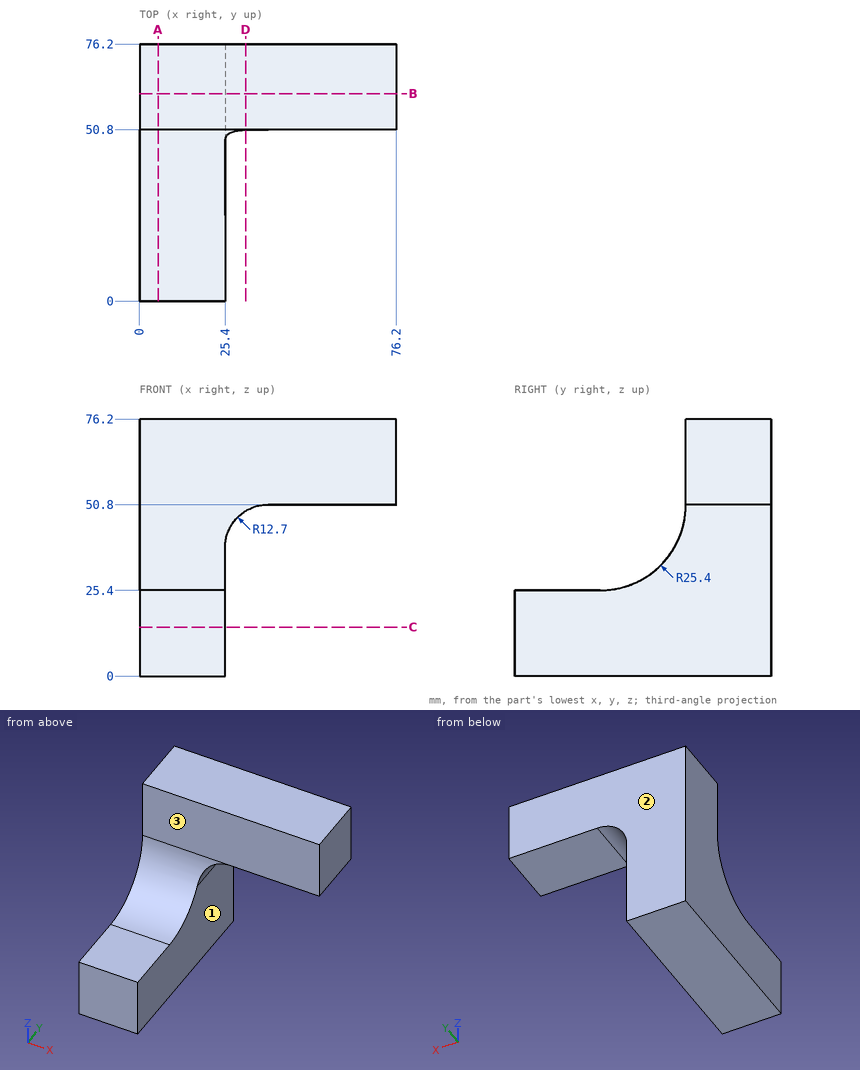
Answer from the drawing. Dimensions are ordinates in mm from the lowest x, y and z of the part. A direction names the side the tool comes from. Give positions to 0.01 mm unless a question says otherwise; leave off trailing zeros. Order: outer loops, then holes, each group sorted by start corner. A loop starts at its lowest first (then second) coordinate and runs counter-clockwise, first axis right, second up.
(1) Find section A-A (x = 5.5). Give the vertices of the cut face in (y, z), plus the area to 3 significant figures.
(2) For the marked faces 1, 2 and 3, determine the directions among +Z, -Z, +X, -X, +Y, -Y from which every point of the face is accessible in a straight line to the end or side of a thin tool.
(3) Find section B-B (y = 61.5). Give the vertices of the cut face in (x, z), plus the area to 3 significant figures.
(4) Given pin 1 (7.5 mm diameter, centred on x = 50.5, y = 67, fed in from -Z); pin 2 (12.5 mm diameter, centred on x = 36.5, z = 66, fed in from -Y); pin 3 (1.5 mm diameter, centred on x = 17.5, y = 45, fed in from +Z), each flat-ended and moving along its own axis, determine where each tip first touches the part or whether it passes through.
(5) Straight lines are drawn through the part: L1, parallel to X at y = 10, z = 6; L2, parallel to Z at x = 60.5, y = 64.5. For each, find the intervals that lie inside material, in ascending order.
(6) Find section C-C (z = 14.5). Give the vertices of the cut face in (x, y).
(7) Find section D-D (x = 31.5). Give the vertices of the cut face in (y, z), plus the area to 3 significant figures.
Result sheet:
1. outline: (0, 0) - (76.2, 0) - (76.2, 76.2) - (50.8, 76.2) - (50.8, 50.8) arc R25.4 cw to (25.4, 25.4) - (0, 25.4) - close
1. area: 3,360 mm2
2. face 1: -Z, +X, +Y, -Y
2. face 2: +Z, -Z, +X, -X, +Y
2. face 3: +Z, +X, -X, -Y
3. outline: (0, 0) - (25.4, 0) - (25.4, 38.1) arc R12.7 cw to (38.1, 50.8) - (76.2, 50.8) - (76.2, 76.2) - (0, 76.2) - close
3. area: 3,260 mm2
4. pin 1: stops at z = 50.8
4. pin 2: stops at y = 50.8
4. pin 3: stops at z = 35.6
5. L1: x = 0 to 25.4
5. L2: z = 50.8 to 76.2
6. outline: (0, 0) - (25.4, 0) - (25.4, 76.2) - (0, 76.2) - close
7. outline: (50.73, 48.95) - (76.2, 48.95) - (76.2, 76.2) - (50.8, 76.2) - (50.8, 50.8) arc R25.4 cw to start
7. area: 692 mm2
